Here's how the part is built. I have some questions about the finished solid (model axes, mm). A direction names the side the tool comes from. Give positions to 0.01 mm unless a question says otherwise; leave off trailing zeros. Loops run counter-clockwise (first coordinate to the right, second up) from the corner with the lowest first, then second, coordinate; pieces in that order, holes last. Notation, with made-up numbers: (69, -31) -> (83, -31) arc R26 cw to (83, -5) -> close; hole circle Ø3 at (25, 1). An arc over 180 degrees is marked (long way). Answer in a Markdown table with one row per item. Add a question column.
Item 1: If I drill on line 1 (Z direction, x = 240.5, y = -527); line 2 (Z direction, x = 229, y = -263); line 3 (Y direction, x = 570.5, z = -753), over which ranges is the centre line in solid material (lowest first)?
Item 2: We'd pull the mould along Z, two halves only. Please class faces 1 (the face through (-498, -272, -657.848)), 2 (the face through (577, -272, -752.848)), 3 (the face through (-560.184, -279, 19)): released by +Z, released by -Z, zero draft, split by the parting line, or undercut.
Item 3: If we section it at A-A (y = -446.5): Write out the boundary of the cut face in (x, z), then the cut area to 3 significant figures.
Item 4: If we section it at C-C (z = -342.5): Write out the boundary of the cut face in (x, y).
Item 5: If we section it at D-D (z = -48): Write out the boundary of the cut face in (x, y), then the cut area to 3 significant figures.
Item 6: For P1, Ø13.5, axis at y = -520.5, z = -389.5, coming from the +X side; P2, Ø13.5, axis at x = -100.5, y = -523, coming from the -Z side; P3, Ø13.5, axis at x = 566.5, y = -337.5, coming from the -Z side, each with a flat end and sliding along its axis, tell me the tip position at first contact or that it passes through.
Item 7: Which directions (+Z, -Z, +X, -X, +Y, -Y) give clear straight access to the entire face, cutting with the end or side of a thin tool? Please do faces 4 (the face through (-430.184, -22, -799)), 5 (the face through (32, -550, -701)), 6 (the face through (-475.184, -272, -703)), 7 (the face through (33, -22, -657.848)).
Item 8: If we section it at B-B (x = -320): Write out the boundary of the cut face in (y, z).
```python
from build123d import *

# Parameters (mm, degrees)
F0_W      = 940
F0_H      = 90
F1_DEPTH  = 45
F3_W      = 45
F3_H      = 90
F3_H_2    = 95
F4_DEPTH  = 460
F6_W      = 940
F6_H      = 90
F7_DEPTH  = 45
F8_W      = 1200
F8_H      = 606
F9_DEPTH  = 19
F11_W     = 1200
F11_H     = 606
F12_DEPTH = 19


with BuildPart() as f1:
    # F0 (on Front) → F1 (new body)
    with BuildSketch(Plane.XZ):
        with Locations((39.816496, -32.848117)):
            Rectangle(F0_W, F0_H)
        Polygon((-430.183504, -77.848117), (-430.183504, 12.151883), (-520.183504, 12.151883), (-520.183504, -847.848117), (-430.183504, -847.848117), (-430.183504, -747.848117), (-430.183504, -657.848117), align=None)
        Polygon((599.816496, 12.151883), (509.816496, 12.151883), (509.816496, -77.848117), (509.816496, -657.848117), (509.816496, -747.848117), (509.816496, -847.848117), (599.816496, -847.848117), align=None)
        with Locations((39.816496, -702.848117)):
            Rectangle(F0_W, F0_H)
    extrude(amount=F1_DEPTH)

    # F3 (on offset) → F4 (join)
    with BuildSketch(Plane.XZ.offset(45)):
        with Locations((-497.683504, -32.848117)):
            Rectangle(F3_W, F3_H)
        with Locations((577.316496, -32.848117)):
            Rectangle(F3_W, F3_H)
        with Locations((577.316496, -705.348117)):
            Rectangle(F3_W, F3_H_2)
        with Locations((-497.683504, -702.848117)):
            Rectangle(F3_W, F3_H)
    extrude(amount=F4_DEPTH)

    # F6 (on offset) → F7 (join)
    with BuildSketch(Plane.XZ.offset(505)):
        with Locations((39.816496, -32.848117)):
            Rectangle(F6_W, F6_H)
        Polygon((-430.183504, -77.848117), (-430.183504, 12.151883), (-520.183504, 12.151883), (-520.183504, -847.848117), (-430.183504, -847.848117), (-430.183504, -747.848117), (-430.183504, -657.848117), align=None)
        Polygon((599.816496, 12.151883), (509.816496, 12.151883), (509.816496, -77.848117), (509.816496, -657.848117), (509.816496, -747.848117), (509.816496, -847.848117), (599.816496, -847.848117), align=None)
        with Locations((39.816496, -702.848117)):
            Rectangle(F6_W, F6_H)
    extrude(amount=F7_DEPTH)

    # F8 (on Top) → F9 (join)
    with BuildSketch(Plane.XY):
        with Locations((39.816496, -275)):
            Rectangle(F8_W, F8_H)
    extrude(amount=F9_DEPTH)

    # F11 (on offset) → F12 (join)
    with BuildSketch(Plane.XY.offset(19)):
        with Locations((39.816496, -275)):
            Rectangle(F11_W, F11_H)
    extrude(amount=F12_DEPTH)


solid = f1.part
```
Recorded:
| question | item | result |
|---|---|---|
| 1 | line 1 | z = -747.85 to -657.85, -77.85 to 38 |
| 1 | line 2 | z = 0 to 38 |
| 1 | line 3 | y = -550 to -505, -45 to 0 |
| 2 | face 1 | undercut |
| 2 | face 2 | released by -Z |
| 2 | face 3 | zero draft |
| 3 | outline | (-560.18, 0) -> (-520.18, 0) -> (-520.18, -77.85) -> (-475.18, -77.85) -> (-475.18, 0) -> (554.82, 0) -> (554.82, -77.85) -> (599.82, -77.85) -> (599.82, 0) -> (639.82, 0) -> (639.82, 38) -> (-560.18, 38) -> close; (-520.18, -747.85) -> (-475.18, -747.85) -> (-475.18, -657.85) -> (-520.18, -657.85) -> close; (554.82, -752.85) -> (599.82, -752.85) -> (599.82, -657.85) -> (554.82, -657.85) -> close |
| 3 | area | 60,900 mm^2 |
| 4 | outline | (-520.18, -550) -> (-430.18, -550) -> (-430.18, -505) -> (-520.18, -505) -> close; (-520.18, -45) -> (-430.18, -45) -> (-430.18, 0) -> (-520.18, 0) -> close; (509.82, -550) -> (599.82, -550) -> (599.82, -505) -> (509.82, -505) -> close; (509.82, -45) -> (599.82, -45) -> (599.82, 0) -> (509.82, 0) -> close |
| 5 | outline | (-520.18, -550) -> (599.82, -550) -> (599.82, 0) -> (-520.18, 0) -> close; hole (-475.18, -505) -> (554.82, -505) -> (554.82, -45) -> (-475.18, -45) -> close |
| 5 | area | 142,000 mm^2 |
| 6 | P1 | stops at x = 599.82 |
| 6 | P2 | stops at z = -747.85 |
| 6 | P3 | stops at z = -752.85 |
| 7 | face 4 | -Z, +Y, -Y |
| 7 | face 5 | -Z, +X, -X, -Y |
| 7 | face 6 | -Z |
| 7 | face 7 | +Y, -Y |
| 8 | outline | (-578, 0) -> (-550, 0) -> (-550, -77.85) -> (-505, -77.85) -> (-505, 0) -> (-45, 0) -> (-45, -77.85) -> (0, -77.85) -> (0, 0) -> (28, 0) -> (28, 38) -> (-578, 38) -> close; (-550, -747.85) -> (-505, -747.85) -> (-505, -657.85) -> (-550, -657.85) -> close; (-45, -747.85) -> (0, -747.85) -> (0, -657.85) -> (-45, -657.85) -> close |
